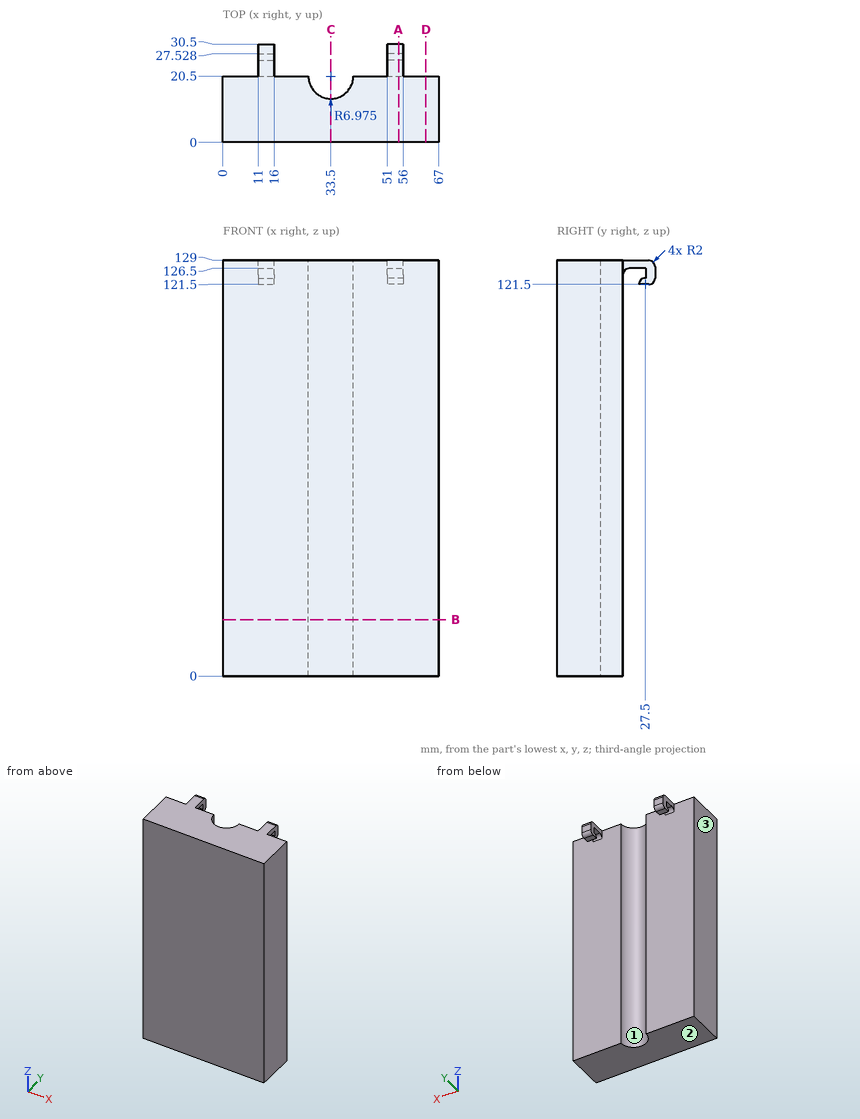
Check sheet for the drawn part. Datum: minimum x, y, z corner. Units: mm. Coordinates: 2 decimals unless noted, no trailing zeros. Order: outer loops, then holes, each group sorted by start corner. A loop starts at its lowest first (then second) coordinate and runs counter-clockwise, first axis right, second up. Notation, with made-up numbers: M 56.5,80 L 93.5,80 A21 ccw 93.5,113 Z; hole C 45.5,51.25 d8. An arc over 180 degrees is marked long. One line per item, written item: value. Start each with the question number.
Item 1: Gauge pin test, flat ends, axial feed: pin 1 (4 mm diameter, centred on y = 26.5, z = 124, fed in from -X); pin 2 (1.5 mm diameter, centred on x = 14.5, y = 27, fed in from -Z); pin 3 (8 mm diameter, centred on y = 27.5, z = 125.5, fed in from +X). Record the tip position at first contact, or that the pin passes through.
Item 2: Sectioned sample at A-A (x = 54.5). Enter the section's corners in (y, z).
Item 3: Mould release check, pull along X, two halves, no side actions. Record for the marked faces 1, 2 and 3: released by +X, released by -X, zero draft, split by the parting line, or undercut.
Item 4: Scan lines: probe 1 along Y at (x, z) = (15, 40); probe 2 along X at (y, z) = (16, 84.5); probe 3 along Y at (x, z) = (33, 23). Record each from-to range of solid material in increasing order.
Item 5: Sectioned sample at B-B (z = 17.5). Enter the section's corners in (x, y) (3 decimals).
Item 6: Sectioned sample at D-D (x = 63). Enter the section's corners in (y, z).
Item 7: Sectioned sample at C-C (x = 33.5). Enter the section's corners in (y, z) (3 decimals), then the cut area to 3 significant figures.
Conclusion:
1. pin 1: stops at x = 11
1. pin 2: stops at z = 121.5
1. pin 3: stops at x = 56
2. outline: M 0,0 L 20.5,0 L 20.5,124.5 A2 cw 22.5,126.5 L 27.53,126.5 L 27.53,123.5 A2 ccw 25.5,121.5 L 28.5,121.5 A2 ccw 30.5,123.5 L 30.5,127 A2 ccw 28.5,129 L 0,129 Z
3. face 1: undercut
3. face 2: zero draft
3. face 3: released by -X
4. probe 1: y = 0 to 20.5
4. probe 2: x = 0 to 28.17, 38.83 to 67
4. probe 3: y = 0 to 13.54
5. outline: M 0,0 L 67,0 L 67,20.5 L 40.475,20.5 A6.975 cw 26.525,20.5 L 0,20.5 Z
6. outline: M 0,0 L 20.5,0 L 20.5,129 L 0,129 Z
7. outline: M 0,0 L 13.525,0 L 13.525,129 L 0,129 Z
7. area: 1,740 mm^2
